from build123d import *

# Parameters (mm, degrees)
F0_R     = 18
F0_R_2   = 13.6738896343
F2_DEPTH = 7
F1_R     = 13.7073607276
F3_DEPTH = 8
F4_R     = 1


# Not quite as in the source:
# - a fillet or chamfer that OpenCascade refuses, or shapes differently, is made with other operations: its cross-section is extruded or revolved along the edge and cut away or added


with BuildPart() as f2:
    # F0 (on Front) → F2 (new body)
    with BuildSketch(Plane.XZ):
        Circle(F0_R)
        Circle(F0_R_2, mode=Mode.SUBTRACT)
    extrude(amount=-F2_DEPTH)

    # F1 (on Front) → F3 (join)
    with BuildSketch(Plane.XZ):
        Circle(F1_R)
    extrude(amount=-F3_DEPTH)

    # F4
    f4_edges = [f2.edges().sort_by_distance(p)[0] for p in [
        (18, 3.5, 0),
        (-18, 0, 0),
        (-18, 7, 0),
    ]]
    fillet(f4_edges, radius=F4_R)

    # F5: fillet of radius 90 on 1 edges, made by hand

    # F5_s1 → F5_t2 (revolve, cut)
    with BuildSketch(Plane.XY):
        with BuildLine():
            ThreePointArc((13.7073607276, 7), (7.0364764999, 7.7496518099), (0.3282725674, 8))
            Line((0.3282725674, 8), (13.7073607276, 8))
            Line((13.7073607276, 8), (13.7073607276, 7))
        make_face()
    revolve(axis=Axis((0, 8, 0), (0, -1, 0)), mode=Mode.SUBTRACT)


solid = f2.part
Could you check a few things on this model? Use its own coordinates, in mm. A direction names the side the tool comes from. Coordinates: 2 decimals unless noted, no trailing zeros. Loops run counter-clockwise (first coordinate to the right, second up) from the corner with the lowest first, then second, coordinate; pieces in that order, holes last. Notation, with made-up numbers: (-1, 86.5) -> (37, 86.5) arc R16 ccw to (37, 103.5) -> close; hole circle Ø1 at (37, 0). An arc over 180 degrees is marked (long way). Answer in a Markdown table with one row per item.
(1) Imagine slicing it at A-A (y = 1.75). List the corners of the cut face in (x, z) for me.
Results found:
| item | result |
|---|---|
| outline | circle Ø36 at (0, 0) |
(2) If I drill on probe 1 along Z at (x, y) = (-0.5, 3.75); probe 2 along Y at (x, z) = (-1.5, 0.5), over which ranges is the centre line in solid material (lowest first)?
Results found:
| item | result |
|---|---|
| probe 1 | z = -17.99 to 17.99 |
| probe 2 | y = 0 to 7.99 |
(3) Will these pins go through, and if not, where does the flat tip stop? pin 1 Ø1.5 at (y, z) = (6, -4.5) entering from +X; pin 2 Ø1.5 at (x, z) = (-1, -13) entering from +Y; pin 3 Ø1 at (x, z) = (-10.5, -5.5) entering from +Y.
Results found:
| item | result |
|---|---|
| pin 1 | stops at x = 17.61 |
| pin 2 | stops at y = 7.2 |
| pin 3 | stops at y = 7.32 |
(4) Imagine slicing it at B-B (y = 6.5). List the corners of the cut face in (x, z) for me.
Results found:
| item | result |
|---|---|
| outline | circle Ø35.73 at (0, 0) |
(5) For faces 1 (the face through (1, 7, 14)), 2 (the face through (-2.343, 3.465, 17.847)), which set-ups out of +Z, -Z, +X, -X, +Y, -Y let a thin tool reach every point of the face, with its end or its side?
Results found:
| item | result |
|---|---|
| face 1 | +Y |
| face 2 | +Y, -Y |
